The listing builds one solid part. Answer for the finished solid, in the listing's coordinates (mm). A direction names the side the tool comes from. Round coordinates to 2 decimals unless told otherwise and drop trailing zeros. Order: outer loops, then holes, each group sorted by start corner. A loop starts at its lowest first (then second) coordinate and runs counter-clockwise, first axis right, second up. Notation, with made-up numbers: (19.25, -11) -> (34.25, -11) arc R25 ccw to (34.25, 6) -> close; hole circle Ø3 at (18.5, 29.5). An arc over 180 degrees is marked (long way). Return JSON: item names as keys, results as strings. Group by question number.
(1) Determine the mould class of faces 1 (the face through (-1, 5, -41.2)), 2 (the face through (-1, 5, 42.635)), 3 (the face through (-65, 9, 0)) for opening direction Z: +Z half, -Z half, draft (parallel to the pull), parting line (faces both ways), or undercut.
(2) Which of the six approach directions +Z, -Z, +X, -X, +Y, -Y give full straight-line access (tool end or side, diameter ignored) to faces 4 (the face through (-1, 5, -42.635)), 5 (the face through (65, 9, 0)), 6 (the face through (-1, 5, 41.2))?
(3) Each of these flat-tipped pins is pushed along its axis until it touches: pin 1 (0.9 mm diameter, centred on x = 66, z = 0, fed in from -Y); pin 2 (3 mm diameter, centred on y = 6, z = -3, fed in from -X); pin 3 (0.5 mm diameter, centred on x = 66.5, y = 9.5, fed in from +Z); pin 4 (3.5 mm diameter, centred on x = -64.5, z = -0.5, fed in from -Y). Where does it stop, or does it pass through?
(4) Consider line 1 (Z direction, x = 58.5, y = 3.75) (3 decimals); line 2 (X direction, y = 9.75, z = 25). Determine where each line is inside the solid, lowest interval first. Write a range as [from, to].
(5) The part is cut by section B-B (z = -13). Determine the outline of the cut face in (x, y), plus the area to 4 significant figures.
(6) The part is cut by section A-A (y = 5.5). Determine the outline of the cut face in (x, z) (3 decimals).
(7) The part is cut by section C-C (x = -39.5). Determine the outline of the cut face in (y, z) (3 decimals), plus the area to 4 significant figures.
from build123d import *

# Parameters (mm, degrees)
SKETCH2_W           = 127.56
SKETCH2_H           = 85.27
SKETCH2_W_2         = 124.2
SKETCH2_H_2         = 82.4
BOSS_EXTRUDE1_DEPTH = 10
SKETCH3_W           = 8
SKETCH3_H           = 1
BOSS_EXTRUDE2_DEPTH = 3
CHAMFER1_SIZE       = 0.5
FILLET1_R           = 2


with BuildPart() as part:
    # Sketch2 → Boss-Extrude1 (new body)
    with BuildSketch(Plane(origin=(0, 0, 0), x_dir=(1, 0, 0), z_dir=(0, 1, 0))):
        Rectangle(SKETCH2_W, SKETCH2_H)
        Rectangle(SKETCH2_W_2, SKETCH2_H_2, mode=Mode.SUBTRACT)
    extrude(amount=BOSS_EXTRUDE1_DEPTH)

    # Sketch3 → Boss-Extrude2 (add)
    with BuildSketch(Plane.ZY.offset(63.78)):
        with Locations((0, 9.5)):
            Rectangle(SKETCH3_W, SKETCH3_H)
    boss_extrude2 = extrude(amount=BOSS_EXTRUDE2_DEPTH)

    # Chamfer1
    chamfer1_edges = [part.edges().sort_by_distance(p)[0] for p in [
        (0, 0, 42.635),
        (-63.78, 0, 0),
        (0, 0, -42.635),
        (63.78, 0, 0),
    ]]
    chamfer(chamfer1_edges, length=CHAMFER1_SIZE)

    # Mirror1: Boss-Extrude2 across plane
    add(boss_extrude2.mirror(Plane(origin=(0, 0, 0), x_dir=(0, 0, 1), z_dir=(1, 0, 0))))

    # Fillet1
    fillet1_edges = [part.edges().sort_by_distance(p)[0] for p in [
        (-63.78, 9.5, -4),
        (-63.78, 9.5, 4),
        (63.78, 9.5, -4),
        (63.78, 9.5, 4),
    ]]
    fillet(fillet1_edges, radius=FILLET1_R)


solid = part.part
Answer below:
{
 "1": {"face 1": "undercut", "face 2": "+Z half", "face 3": "draft"},
 "2": {"face 4": "-Z, +X, -X, +Y, -Y", "face 5": "+Z, -Z, +X, -Y", "face 6": "+Y, -Y"},
 "3": {"pin 1": "stops at y = 9", "pin 2": "stops at x = -63.78", "pin 3": "stops at z = 4", "pin 4": "stops at y = 0"},
 "4": {"line 1": "z = [-42.635, -41.2], [41.2, 42.635]", "line 2": "x = [-63.78, -62.1], [62.1, 63.78]"},
 "5": {"outline": "(-63.78, 0.5) -> (-63.28, 0) -> (-62.1, 0) -> (-62.1, 10) -> (-63.78, 10) -> close; (62.1, 0) -> (63.28, 0) -> (63.78, 0.5) -> (63.78, 10) -> (62.1, 10) -> close", "area": "33.35 mm²"},
 "6": {"outline": "(-63.78, -42.635) -> (63.78, -42.635) -> (63.78, 42.635) -> (-63.78, 42.635) -> close; hole (-62.1, -41.2) -> (62.1, -41.2) -> (62.1, 41.2) -> (-62.1, 41.2) -> close"},
 "7": {"outline": "(0, -42.135) -> (0.5, -42.635) -> (10, -42.635) -> (10, -41.2) -> (0, -41.2) -> close; (0, 41.2) -> (10, 41.2) -> (10, 42.635) -> (0.5, 42.635) -> (0, 42.135) -> close", "area": "28.45 mm²"}
}
